Here's how the part is built. I have some questions about the finished solid (model axes, mm). Round coordinates to 2 decimals unless told otherwise and drop trailing zeros. Order: outer loops, then holes, each group sorted by start corner. A loop starts at its lowest first (then second) coordinate and runs counter-clockwise, first axis right, second up. Notation, with made-up numbers: (57, 36) - (98, 36) arc R24 cw to (98, 46) - close; hole circle Ø5 at (72.25, -21.75). An arc over 180 degrees is marked (long way). One line per item, written item: value.
Autodesk Fusion 360 part; units mm, degrees
sketch "Sketch1" plane through (0, 0, 0) normal (1, 0, 0) x (0, 1, 0)
  line L0 (25, 0) -> (25, 150)
  line L1 (25, 150) -> (50, 150)
  line L2 (50, 150) -> (50, 130)
  line L3 (50, 130) -> (28, 130)
  line L4 (28, 130) -> (28, 42)
  line L5 (28, 42) -> (50, 20)
  line L6 (50, 20) -> (50, 0)
  line L7 (50, 0) -> (25, 0)
  line L8 (0, 0) -> (0, 146.3043) construction
  dimension "d1" = 3
  dimension "d2" = 25
  dimension "d3" = 150
  dimension "d4" = 50
  dimension "d5" = 20
  dimension "d6" = 20
  dimension "d7" = 135
revolve "Revolve1" add sketch "Sketch1" angle 360 about axis through (0, 0, 0) along (0, 0, 1)
sketch "Sketch2" plane through (0, 0, 150) normal (0, 0, 1) x (-1, 0, 0)
  circle A0 centre (0, 0) radius 25
  circle A1 centre (0, 0) radius 50
  line L0 (0, 0) -> (-29.3893, 40.4508) construction
  line L1 (0, 0) -> (0, 50) construction
  arc A2 (-1.5, 27.9598) -> (-15.2208, 23.5016) centre (0, 0) ccw
  arc A3 (-1.5, 46.9761) -> (-26.3983, 38.8861) centre (0, 0) ccw
  line L2 (-1.5, 27.9598) -> (-1.5, 46.9761)
  line L3 (-15.2208, 23.5016) -> (-26.3983, 38.8861)
  dimension "d9" = 36
  dimension "d10" = 1.5
  dimension "d11" = 1.5
  dimension "d12" = 3
  dimension "d13" = 3
extrude "Extrude1" cut sketch "Sketch2" against normal up to surface (150 mm away) contours A2 A3 L2 L3
pattern_circular "C-Pattern1" count 10 over 360 about axis through (0, 0, 150) along (0, 0, -1) of "Extrude1"
Q1. If we section it at A-A, the plane z = 85.5: Please give me the cut outline in (x, y), then the cut area to 3 significant figures.
Results list:
outline: circle Ø56 at (0, 0); hole circle Ø50 at (0, 0)
area: 500 mm²
Q2. If we section it at B-B, the plane x = 41: Give the number of separate pieces and of enclosed holes in the cut face, then the cut area to 3 significant figures.
Results list:
separate pieces: 8
enclosed holes: 0
area: 764 mm²
Q3. If I drill on line 1 along Y through (x, z) = (0, 111.5); line 2 along Y through (x, z) = (11, 7.5) (3 decimals); line 3 along Y through (x, z) = (-10, 8.5), over which ranges is the centre line in solid material (lowest first)?
Results list:
line 1: -28 to -25, 25 to 28
line 2: -48.775 to -45.695, -25.749 to -22.45, 22.45 to 25.749, 45.695 to 48.775
line 3: -48.99 to -45.92, -26.15 to -22.91, 22.91 to 26.15, 45.92 to 48.99
Q4. Will these pins go through, and if not, where does the flat tip stop? pin 1 (9.5 mm diameter, centred on y = -37.5, z = 17, fed in from -X); pin 2 (15 mm diameter, centred on y = 40.5, z = 140, fed in from +X); pin 3 (1.5 mm diameter, centred on x = 18, z = 30.5, fed in from +Y).
Results list:
pin 1: x = -37.78
pin 2: x = 37.56
pin 3: y = 28.36
